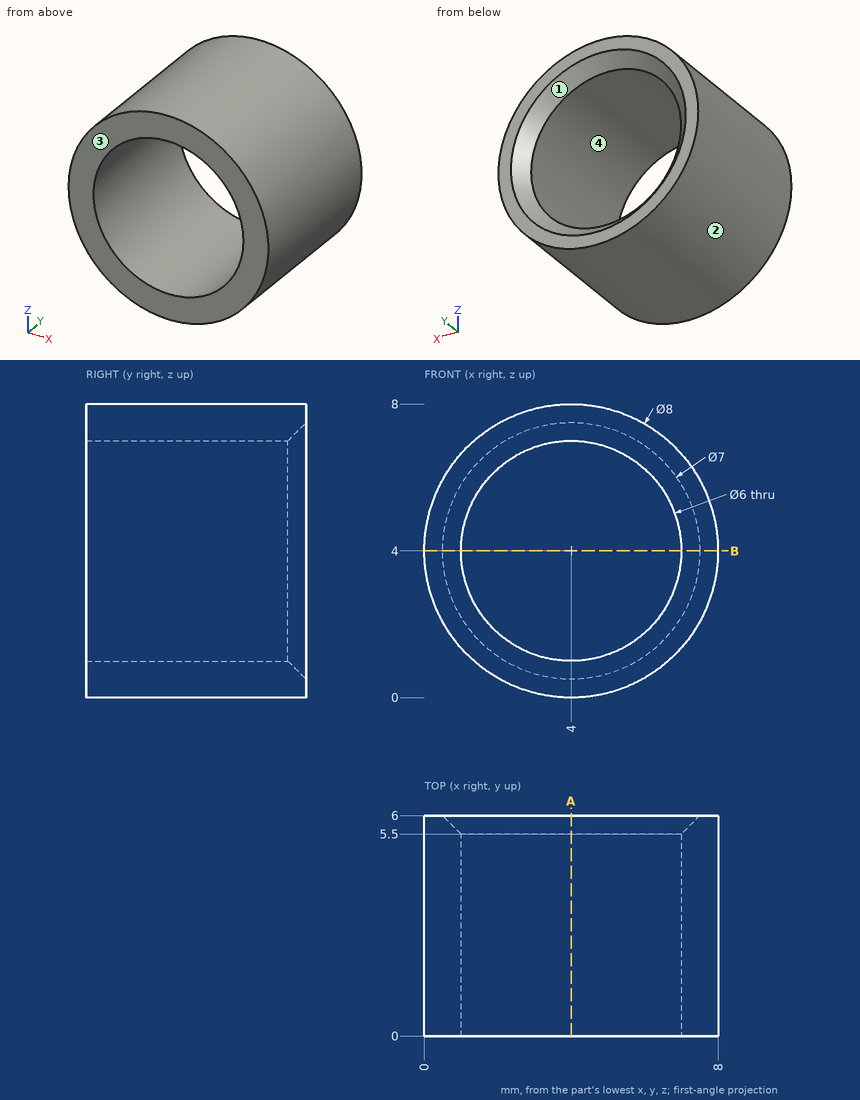
Geometry: see drawing. Coordinates: mm, zero at the bounding-box minimum. Coordinates: 2 decimals unless noted, no trailing zeros. Order: outer loops, then holes, each group sorted by start corner. A loop starts at its lowest first (then second) coordinate and runs counter-clockwise, first axis right, second up. Notation, with made-up numbers: M -11.5,5 L 18.5,5 A18 ccw 18.5,10 Z; hole C 25.5,17 d10. An arc over 180 degrees is marked long. Answer in a Markdown table with one row per item. Add a question column.
Q1. Section query A-A on x = 4. Return the cut outline in (y, z).
Q2. Line query: L1, parallel to Z at x = 4, y = 3.2; L2, parallel to X at y = 0.6, z = 6.75; L3, parallel to Z at x = 3.25, y = 1.05. Output: solid intervals per line, ascending.
Q3. Mould query, pull axis Z, two halves, no side actions, for the marked faces 1, 2, 3 and 4. Classes: released by +Z, released by -Z, zero draft, split by the parting line, or undercut.
Q4. Section query B-B on z = 4. Return the cut outline in (x, y), and give its area (4 significant figures).
Q5. Contact query for flat-ended pins moving along their axis: P1, Ø3, axis at y = 1, z = 2, coming from the +X side; P2, Ø1, axis at x = 3, y = 1, coming from the -Z side; P3, Ø3, axis at x = 6, y = 3, coming from the +Z side. Output: stop coordinate, or through.
Completed:
| question | item | result |
|---|---|---|
| 1 | outline | M 0,0 L 6,0 L 6,0.5 L 5.5,1 L 0,1 Z; M 0,7 L 5.5,7 L 6,7.5 L 6,8 L 0,8 Z |
| 2 | L1 | z = 0 to 1, 7 to 8 |
| 2 | L2 | x = 1.1 to 2.8, 5.2 to 6.9 |
| 2 | L3 | z = 0.07 to 1.1, 6.9 to 7.93 |
| 3 | face 1 | undercut |
| 3 | face 2 | split by the parting line |
| 3 | face 3 | zero draft |
| 3 | face 4 | undercut |
| 4 | outline | M 0,0 L 1,0 L 1,5.5 L 0.5,6 L 0,6 Z; M 7,0 L 8,0 L 8,6 L 7.5,6 L 7,5.5 Z |
| 4 | area | 11.75 mm2 |
| 5 | P1 | stops at x = 7.97 |
| 5 | P2 | stops at z = 0.03 |
| 5 | P3 | stops at z = 7.97 |
